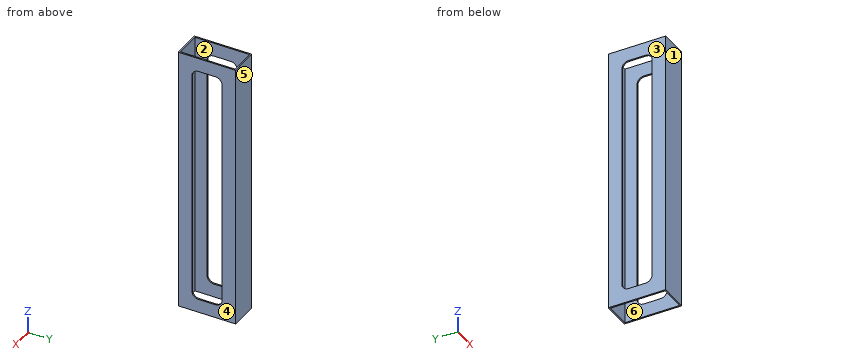
```python
from build123d import *

# Parameters (mm, degrees)
SKETCH1_W           = 25.4
SKETCH1_H           = 50.8
SKETCH1_W_2         = 22.86
SKETCH1_H_2         = 48.26
BOSS_EXTRUDE1_DEPTH = 237.2995
CUT_EXTRUDE5_DEPTH  = 26.4


with BuildPart() as part:
    # Sketch1 → Boss-Extrude1 (new body)
    with BuildSketch(Plane.XY):
        with Locations((-102.657065342, -11.879495554)):
            Rectangle(SKETCH1_W, SKETCH1_H)
        with Locations((-102.657065342, -11.879495554)):
            Rectangle(SKETCH1_W_2, SKETCH1_H_2, mode=Mode.SUBTRACT)
    extrude(amount=BOSS_EXTRUDE1_DEPTH)

    # Sketch4 → Cut-Extrude5 (cut, through all)
    with BuildSketch(Plane(origin=(-89.957065342, 0, 0), x_dir=(0, 0, -1), z_dir=(1, 0, 0))):
        with BuildLine():
            Line((-18, 1.520504446), (-219.2995, 1.520504446))
            ThreePointArc((-219.2995, 1.520504446), (-223.542140687, -0.236854867), (-225.2995, -4.479495554))
            Line((-225.2995, -4.479495554), (-225.2995, -19.279495554))
            ThreePointArc((-225.2995, -19.279495554), (-223.542140687, -23.522136241), (-219.2995, -25.279495554))
            Line((-219.2995, -25.279495554), (-18, -25.279495554))
            ThreePointArc((-18, -25.279495554), (-13.757359313, -23.522136241), (-12, -19.279495554))
            Line((-12, -19.279495554), (-12, -4.479495554))
            ThreePointArc((-12, -4.479495554), (-13.757359313, -0.236854867), (-18, 1.520504446))
        make_face()
    extrude(amount=-CUT_EXTRUDE5_DEPTH, mode=Mode.SUBTRACT)


solid = part.part
```
Here's how the part is built. I have some questions about the finished solid (model axes, mm). Face numbers are marked on the shaded views. A direction names the side the tool comes from. Coordinates: 2 decimals unless noted, no trailing zeros. Order: outer loops, then holes, each group sorted by start corner. A loop starts at its lowest first (then second) coordinate and runs counter-clockwise, first axis right, second up.
1) Which directions (+Z, -Z, +X, -X, +Y, -Y) give clear straight access to the entire face, cutting with the end or side of a thin tool? Please do the marked faces 5 and 6.
2) Imagine slicing it at D-D on x = -94.25. List the corners of the cut face in (y, z) for me, and give its area (3 significant figures).
3) Imagine slicing it at A-A on y = -33.5. List the corners of the cut face in (x, z) for me.
4) Will these pins go through, and if not, where does the flat tip stop? pin 1 (12 mm diameter, centred on x = -105, y = -5, fed in from -Z); pin 2 (1 mm diameter, centred on x = -90.5, y = -8.5, fed in from -Z).
5) Imagine slicing it at C-C on z = 161. List the corners of the cut face in (x, y) for me.
6) Imagine slicing it at B-B on y = -17. List the corners of the cut face in (x, z) for me, and give its area (3 significant figures).
7) We'd pull the mould along X, two halves only. Please class the marked faces 1, 2, 3 and 4: +X half, -X half, draft (parallel to the pull), parting line (faces both ways), or undercut.
8) I need wall thicknesses on line 1 (Y direction, x = -104.75, z = 117); line 2 (X direction, y = 7.5, z = 20). Which ranges of each line are inside material? Lowest first, please.
Response values:
1. face 5: +Z, -Z, +X, -X, +Y
1. face 6: +Z, -Z
2. outline: (-37.28, 0) - (-36.01, 0) - (-36.01, 237.3) - (-37.28, 237.3) - close; (12.25, 0) - (13.52, 0) - (13.52, 237.3) - (12.25, 237.3) - close
2. area: 603 mm2
3. outline: (-115.36, 0) - (-114.09, 0) - (-114.09, 237.3) - (-115.36, 237.3) - close; (-91.23, 0) - (-89.96, 0) - (-89.96, 237.3) - (-91.23, 237.3) - close
4. pin 1: passes through
4. pin 2: stops at z = 0
5. outline: (-115.36, -37.28) - (-89.96, -37.28) - (-89.96, -25.28) - (-91.23, -25.28) - (-91.23, -36.01) - (-114.09, -36.01) - (-114.09, -25.28) - (-115.36, -25.28) - close; (-115.36, 1.52) - (-114.09, 1.52) - (-114.09, 12.25) - (-91.23, 12.25) - (-91.23, 1.52) - (-89.96, 1.52) - (-89.96, 13.52) - (-115.36, 13.52) - close
6. outline: (-115.36, 0) - (-114.09, 0) - (-114.09, 12) - (-115.36, 12) - close; (-115.36, 225.3) - (-114.09, 225.3) - (-114.09, 237.3) - (-115.36, 237.3) - close; (-91.23, 0) - (-89.96, 0) - (-89.96, 12) - (-91.23, 12) - close; (-91.23, 225.3) - (-89.96, 225.3) - (-89.96, 237.3) - (-91.23, 237.3) - close
6. area: 61.0 mm2
7. face 1: draft
7. face 2: undercut
7. face 3: -X half
7. face 4: +X half
8. line 1: y = -37.28 to -36.01, 12.25 to 13.52
8. line 2: x = -115.36 to -114.09, -91.23 to -89.96
